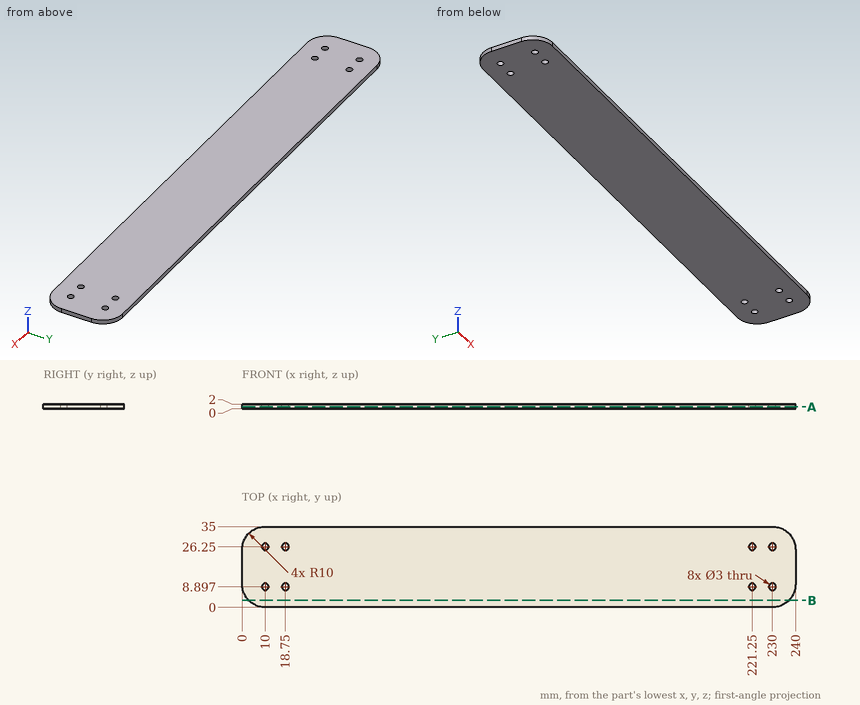
Verification items for this drawing (mm, ordinates from the low corner). Give positions to 0.01 mm unless a question says otherwise; leave off trailing zeros. Loops run counter-clockwise (first coordinate to the right, second up) from the corner with the lowest first, then second, coordinate; pieces in that order, holes last. Notation, with made-up numbers: M -2.5,34.25 L 28.5,34.25 A16 cw 28.5,54.25 Z; hole C 71,70.25 d3. An arc over 180 degrees is marked long. Write item = value, one per line.
(1) Sectioned sample at A-A, the plane z = 0.8. State how many separate pieces and enclosed holes the cut face has, plus the area to 3 significant figures.
Answer below:
separate_pieces = 1
enclosed_holes = 8
area = 8,260 mm2
(2) Sectioned sample at B-B, the plane y = 3. Record the cut outline in (x, z).
Answer below:
outline = M 2.86,0 L 237.14,0 L 237.14,2 L 2.86,2 Z
(3) Material ranges on line 1 (Y direction, x = 10, z = 1); line 2 (X direction, y = 26.5, z = 1.65); line 3 (X direction, y = 4, z = 1.1), recorded low to high. Write a range as [from, to].
Answer below:
line_1 = [0, 7.4], [10.4, 24.75], [27.75, 35]
line_2 = [0.11, 8.52], [11.48, 17.27], [20.23, 219.77], [222.73, 228.52], [231.48, 239.89]
line_3 = [2, 238]
(4) Gauge pin test, flat ends, axial feed: pin 1 Ø2.5 at (x, y) = (18.75, 26.25) entering from +Z; pin 2 Ø3.5 at (x, y) = (10, 8.9) entering from +Z. Record the tip position at first contact, or that the pin passes through.
Answer below:
pin_1 = through
pin_2 = 2
